The model under review builds one solid part; all positions refer to its coordinate system, in mm. A direction names the side the tool comes from. Round coordinates to 2 decimals unless told otherwise and drop trailing zeros. Write each loop counter-clockwise with the first axis right and the second up, starting at its lowest first coordinate (ties: lowest second). Pieces come first, ordered by that corner, then holes. Notation, with made-up numbers: M 74.5,50.5 L 101.5,50.5 A30 ccw 101.5,72.5 Z; hole C 4,-22.5 d10. An arc over 180 degrees is marked long. One line per item, written item: value. Start each with the question number.
1) Take a section at B-B, the plane y = 179. Write out the cut boundary in (x, z).
2) Take a section at D-D, the plane y = -214. Write out the cut boundary in (x, z), and give its area (3 significant figures).
3) Take a section at C-C, the plane x = -1101.5. Write out the cut boundary in (y, z), and give its area (3 significant figures).
4) Tool access review of faces 1 (the face through (-977.292, -12, 498)), 2 (the face through (-1382.292, -3, 483)), 3 (the face through (-975.292, -12, 497)), 4 (the face through (-1191.03, -225.99, 510.74)), 5 (the face through (-1381.306, 45.755, 469.406)): name each direction out of +Z, -Z, +X, -X, +Y, -Y from which nothing blocks a thin tool from reaching the whole face with its end or side.
5) Wall thickness on probe 1 along X at (y, z) = (-110, 433); probe 2 along X at (y, z) = (-29, 557); probe 3 along Y at (x, z) = (-1034.5, 479): over which ranges is each line inside the solid? List them lowest first.
6) Take a section at A-A, the plane y = 42. Write out the cut boundary in (x, z), and give its area (3 significant figures).
7) Mouldability with a two-part tool opening along Y and no side actions: class faces 6 (the face through (-1272, -227, 497)), 7 (the face through (-1381.306, -38.245, 469.406)), 8 (the face through (-1233.9, -226, 513.4)) as +Y half, -Y half, draft (parallel to the pull), parting line (faces both ways), or undercut.
8) For P1, Ø0.6, axis at x = -1196, z = 433.5, coming from the -Y side; P2, Ø10, axis at x = -1091.5, y = -153.5, coming from the +Z side; P3, Ø22.5, axis at y = -42, z = 457.48, coming from the -X side; P4, Ø5, axis at x = -1342.49, y = -150.3, coming from the -Z side, all flat-tipped, find the tip position at first contact; note any pin that passes through.
from build123d import *

# Parameters (mm, degrees)
DODANIE_WYCI_GNI_CIE1_DEPTH     = 130
SKORUPA1_T                      = 2
WYTNIJ_WYCI_GNI_CIE1_REACH      = 1414.162
SZKIC6_W                        = 132
SZKIC6_H                        = 206
OTWORY_USTALAJ_CE_12_0MM1_D     = 12
OTWORY_USTALAJ_CE_12_0MM1_DEPTH = 2
SZKIC10_R                       = 12.5
SZKIC10_R_2                     = 22.75
WYTNIJ_WYCI_GNI_CIE2_DEPTH      = 10
SZKIC8_R                        = 10
WYTNIJ_WYCI_GNI_CIE3_DEPTH      = 10
SZKIC11_R                       = 2
WYTNIJ_WYCI_GNI_CIE4_DEPTH      = 10
SZKIC12_R                       = 10.5
WYTNIJ_WYCI_GNI_CIE5_DEPTH      = 10


with BuildPart() as part:
    # Szkic1 → Dodanie-wyciągnięcie1 (new body)
    with BuildSketch(Plane.XY.offset(434.283231707)):
        Polygon((-977.291509632, 225), (-977.291509632, -255), (-1162.291509632, -255), (-1162.291509632, -225), (-1380.291509632, -225), (-1380.291509632, 225), align=None)
    extrude(amount=DODANIE_WYCI_GNI_CIE1_DEPTH)

    # Skorupa1
    skorupa1_openings = [part.faces().sort_by_distance(p)[0] for p in [
        (-1175.554752008, -7.126805778, 564.283231707),
    ]]
    offset(amount=SKORUPA1_T, openings=skorupa1_openings, kind=Kind.INTERSECTION)

    # Szkic6 → Wytnij-wyciągnięcie1 (cut, up to next)
    with BuildSketch(Plane(origin=(0, 0, 432.283231707), x_dir=(-1, 0, 0), z_dir=(0, 0, -1)), mode=Mode.PRIVATE) as wytnij_wyci_gni_cie1_sk1:
        with Locations((1191.291509632, 104)):
            Rectangle(SZKIC6_W, SZKIC6_H)
    wytnij_wyci_gni_cie1_tool1 = extrude(wytnij_wyci_gni_cie1_sk1.sketch, amount=-WYTNIJ_WYCI_GNI_CIE1_REACH, mode=Mode.PRIVATE) & part.part
    add(wytnij_wyci_gni_cie1_tool1.solids().sort_by_distance((-1191.29151, 104, 432.283232))[0], mode=Mode.SUBTRACT)

    # Otwory ustalające Ø12.0mm1
    with Locations(Plane(origin=(-1125.291509632, -257, 447.283231707), x_dir=(0, 0, -1), z_dir=(0, -1, 0))):
        with Locations((0, 0), (0, 40), (0, 80)):
            Hole(OTWORY_USTALAJ_CE_12_0MM1_D / 2, depth=OTWORY_USTALAJ_CE_12_0MM1_DEPTH)

    # Szkic10 → Wytnij-wyciągnięcie2 (cut)
    with BuildSketch(Plane.ZY.offset(1382.291509632)):
        with Locations((457.483231707, 42)):
            Circle(SZKIC10_R)
        with Locations((457.483231707, 0)):
            Circle(SZKIC10_R)
        with Locations((457.483231707, -42)):
            Circle(SZKIC10_R)
        with Locations((511.683231707, -3)):
            Circle(SZKIC10_R_2)
    extrude(amount=-WYTNIJ_WYCI_GNI_CIE2_DEPTH, mode=Mode.SUBTRACT)

    # Szkic8 → Wytnij-wyciągnięcie3 (cut)
    with BuildSketch(Plane.XZ.offset(257)):
        with Locations((-1122.291509632, 508.783231707)):
            Circle(SZKIC8_R)
        with Locations((-1059.291509632, 508.783231707)):
            Circle(SZKIC8_R)
    extrude(amount=-WYTNIJ_WYCI_GNI_CIE3_DEPTH, mode=Mode.SUBTRACT)

    # Szkic11 → Wytnij-wyciągnięcie4 (cut)
    with BuildSketch(Plane(origin=(0, 0, 432.283231707), x_dir=(-1, 0, 0), z_dir=(0, 0, -1))):
        with Locations((1363.891509632, -110.6)):
            Circle(SZKIC11_R)
        with Locations((1342.491509632, -150.3)):
            Circle(SZKIC11_R)
        with Locations((1312.491509632, -150.3)):
            Circle(SZKIC11_R)
        with Locations((1333.891509632, -110.6)):
            Circle(SZKIC11_R)
        with Locations((1282.491509632, -150.3)):
            Circle(SZKIC11_R)
        with Locations((1303.891509632, -110.6)):
            Circle(SZKIC11_R)
    extrude(amount=-WYTNIJ_WYCI_GNI_CIE4_DEPTH, mode=Mode.SUBTRACT)

    # Szkic12 → Wytnij-wyciągnięcie5 (cut)
    with BuildSketch(Plane(origin=(0, -225, 0), x_dir=(1, 0, 0), z_dir=(0, 1, 0))):
        with Locations(Location((-1201.521509632, -510.283231707, 0), (0, 0, 180))):
            Circle(SZKIC12_R)
        with Locations(Location((-1223.871509632, -510.283231707, 0), (0, 0, 180))):
            Circle(SZKIC12_R)
        with BuildLine():
            Line((-1211.196509632, -521.783231707), (-1214.196509632, -521.783231707))
            ThreePointArc((-1214.196509632, -521.783231707), (-1216.446509632, -519.533231707), (-1214.196509632, -517.283231707))
            Line((-1214.196509632, -517.283231707), (-1211.196509632, -517.283231707))
            ThreePointArc((-1211.196509632, -517.283231707), (-1208.946509632, -519.533231707), (-1211.196509632, -521.783231707))
        make_face()
    extrude(amount=-WYTNIJ_WYCI_GNI_CIE5_DEPTH, mode=Mode.SUBTRACT)


solid = part.part
Checked values:
1. outline: M -1382.29,432.28 L -1257.29,432.28 L -1257.29,434.28 L -1380.29,434.28 L -1380.29,564.28 L -1382.29,564.28 Z; M -1125.29,432.28 L -975.29,432.28 L -975.29,564.28 L -977.29,564.28 L -977.29,434.28 L -1125.29,434.28 Z
2. outline: M -1382.29,432.28 L -975.29,432.28 L -975.29,564.28 L -977.29,564.28 L -977.29,434.28 L -1380.29,434.28 L -1380.29,564.28 L -1382.29,564.28 Z
2. area: 1,330 mm2
3. outline: M -257,432.28 L 227,432.28 L 227,564.28 L 225,564.28 L 225,434.28 L -255,434.28 L -255,564.28 L -257,564.28 Z
3. area: 1,490 mm2
4. face 1: +Z
4. face 2: +Z, -Z, -X, +Y, -Y
4. face 3: +Z, -Z, +X, +Y, -Y
4. face 4: -Y
4. face 5: -X
5. probe 1: x = -1382.29 to -1365.8, -1361.98 to -1335.8, -1331.98 to -1305.8, -1301.98 to -975.29
5. probe 2: x = -1382.29 to -1380.29, -977.29 to -975.29
5. probe 3: y = -257 to -255, 225 to 227
6. outline: M -1382.29,432.28 L -1257.29,432.28 L -1257.29,434.28 L -1380.29,434.28 L -1380.29,444.98 L -1382.29,444.98 Z; M -1382.29,469.98 L -1380.29,469.98 L -1380.29,564.28 L -1382.29,564.28 Z; M -1125.29,432.28 L -975.29,432.28 L -975.29,564.28 L -977.29,564.28 L -977.29,434.28 L -1125.29,434.28 Z
6. area: 1,020 mm2
7. face 6: -Y half
7. face 7: undercut
7. face 8: draft
8. P1: stops at y = -227
8. P2: stops at z = 434.28
8. P3: stops at x = -977.29
8. P4: stops at z = 432.28
